Geometry check sheet. Reference: the model listing, model coordinates, mm. A direction names the side the tool comes from. Give positions to 0.01 mm unless a question says otherwise; leave off trailing zeros. Loops run counter-clockwise (first coordinate to the right, second up) from the corner with the lowest first, then second, coordinate; pieces in that order, holes last. Notation, with made-up numbers: (3, 8.5) -> (34, 8.5) arc R23 ccw to (34, 32.5) -> close; hole circle Ø11 at (38, 46). An arc over 180 degrees is marked (long way). Write each question's results on one line, items separated by ' | '. Start each with the question number.
1) Depth check by flat-ended pin: pin 1 (1.2 mm diameter, centred on x = -57.5, z = 2.5, fed in from +Y); pin 2 (1.2 mm diameter, centred on y = 109.5, z = 2, fed in from -X); pin 3 (12 mm diameter, centred on x = -72.5, y = 14, fed in from -Z). Enter the tip coordinate at first touch or a pass-through.
2) Sectioned sample at C-C on x = -94. Record the cut outline in (y, z).
3) Scan lines: line 1 (Z direction, x = -5, y = 54); line 2 (Y direction, x = -44, z = 3.75); line 3 (X direction, y = 55, z = 1.85). Record each from-to range of solid material in increasing order. Write a range as from..to.
4) Sectioned sample at A-A on z = 1.2. Record the cut outline in (x, y), then the cut area to 3 significant figures.
5) Sectioned sample at B-B on y = 78.5. Record the cut outline in (x, z).
6) Set-up check for faces 1 (the face through (-5.878, 74, 2)), 2 (the face through (-2.491, 137.986, -0.493)), 3 (the face through (-57, -4.544, 2)): record each of +Z, -Z, +X, -X, +Y, -Y from which the full face is reachable in a straight line by a thin tool's end or side.
```python
from build123d import *

# Parameters (mm, degrees)
SKETCH_1_W      = 10
SKETCH_1_H      = 150
EXTRUDE_1_DEPTH = 4
SKETCH_2_W      = 110
SKETCH_2_H      = 10
EXTRUDE_2_DEPTH = 4
SKETCH_3_R      = 3
EXTRUDE_3_DEPTH = 1


with BuildPart() as part:
    # 草图1 → 凸台-拉伸1 (new body)
    with BuildSketch(Plane.XY):
        with Locations((-0.878378378, 70.456081081)):
            Rectangle(SKETCH_1_W, SKETCH_1_H)
    extrude(amount=EXTRUDE_1_DEPTH)

    # 草图2 → 凸台-拉伸2 (add)
    with BuildSketch(Plane.XY.offset(4)):
        with Locations((-60.878378378, 0.456081081)):
            Rectangle(SKETCH_2_W, SKETCH_2_H)
    extrude(amount=-EXTRUDE_2_DEPTH)

    # 草图3 → 凸台-拉伸3 (add)
    with BuildSketch(Plane(origin=(0, 0, 0), x_dir=(-1, 0, 0), z_dir=(0, 0, -1))):
        with Locations((0.878378378, 135.456081081)):
            Circle(SKETCH_3_R)
    extrude(amount=EXTRUDE_3_DEPTH)


solid = part.part
```
Result:
1) pin 1: y = 5.46 | pin 2: x = -5.88 | pin 3: through
2) outline: (-4.54, 0) -> (5.46, 0) -> (5.46, 4) -> (-4.54, 4) -> close
3) line 1: 0..4 | line 2: -4.54..5.46 | line 3: -5.88..4.12
4) outline: (-115.88, -4.54) -> (4.12, -4.54) -> (4.12, 145.46) -> (-5.88, 145.46) -> (-5.88, 5.46) -> (-115.88, 5.46) -> close | area: 2,600 mm^2
5) outline: (-5.88, 0) -> (4.12, 0) -> (4.12, 4) -> (-5.88, 4) -> close
6) face 1: +Z, -Z, -X, +Y | face 2: -Z | face 3: +Z, -Z, +X, -X, -Y
